Read the model definition and answer for the solid it produces. Units are mm, in the model's axes. Coordinates: 2 decimals unless noted, no trailing zeros. Write each loop counter-clockwise with the first axis right and the second up, starting at its lowest first coordinate (ties: lowest second). Pieces come first, ordered by that corner, then holes. Notation, with made-up numbers: M 41,-29 L 56,-29 A22 ccw 56,-20 Z; hole C -8.5,36.5 d10. An arc over 180 degrees is marked long. Write item = value, one per line.
from build123d import *

# Parameters (mm, degrees)
SKETCH1_W     = 4.3
SKETCH1_H     = 1.5
CHAMFER1_SIZE = 0.2


with BuildPart() as part:
    # Sketch1 → Revolve1 (revolve)
    with BuildSketch(Plane(origin=(0, 0, 0), x_dir=(1, 0, 0), z_dir=(0, 1, 0))):
        with Locations((6.35, 0)):
            Rectangle(SKETCH1_W, SKETCH1_H)
    revolve(axis=Axis((0, 0, 0), (0, 0, -1)))

    # Chamfer1
    chamfer1_edges = [part.edges().sort_by_distance(p)[0] for p in [
        (-4.2, 0, -0.75),
        (-8.5, 0, -0.75),
        (-8.5, 0, 0.75),
        (-4.2, 0, 0.75),
    ]]
    chamfer(chamfer1_edges, length=CHAMFER1_SIZE)


solid = part.part
Item 1: For a pull along X with two mould halves and no side action, classify faces 1 (the face through (4.57, -7.167, -0.008)), 2 (the face through (-4, 4, 0.75)), 3 (the face through (-0.547, -4.164, -0.008)) as released by +X, released by -X, zero draft, split by the parting line, or undercut.
Worked answers:
face_1 = split by the parting line
face_2 = zero draft
face_3 = undercut
Item 2: A flat-ended cylindrical pin translates along its axis: pin 1 (3 mm diameter, centred on x = -3.5, y = 2.5, fed in from -Z). Find the tip coordinate at first contact, or state that the pin passes through.
Worked answers:
pin_1 = -0.75
Item 3: Find section A-A (y = 0). Determine the outline of the cut face in (x, z).
Worked answers:
outline = M -8.5,-0.55 L -8.3,-0.75 L -4.4,-0.75 L -4.2,-0.55 L -4.2,0.55 L -4.4,0.75 L -8.3,0.75 L -8.5,0.55 Z; M 4.2,-0.55 L 4.4,-0.75 L 8.3,-0.75 L 8.5,-0.55 L 8.5,0.55 L 8.3,0.75 L 4.4,0.75 L 4.2,0.55 Z
Item 4: Find section C-C (z = 0). Determine the outline of the cut face in (x, y).
Worked answers:
outline = C 0,0 d17; hole C 0,0 d8.4
Item 5: Consider line 1 along Y through (x, z) = (0, 0.15); line 2 along X through (y, z) = (1.75, -0.5). Determine where each line is inside the solid, lowest interval first. Write a range as from..to.
Worked answers:
line_1 = -8.5..-4.2, 4.2..8.5
line_2 = -8.32..-3.82, 3.82..8.32
